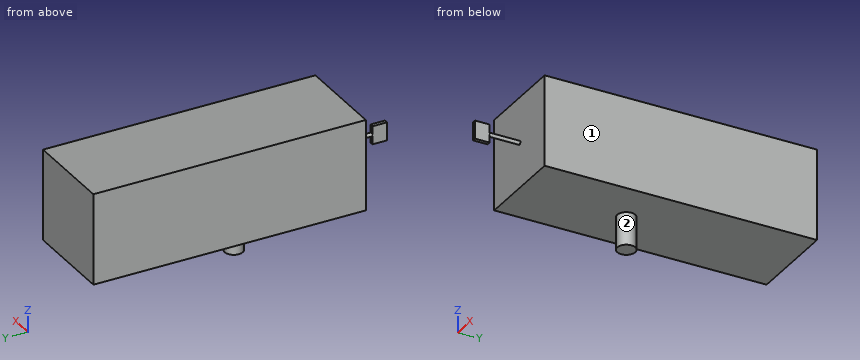
```python
from build123d import *

# Parameters (mm, degrees)
F0_W     = 50
F0_H     = 50
F1_DEPTH = 150
F2_R     = 1
F3_DEPTH = 25
F4_W     = 2
F4_H     = 10
F5_DEPTH = 8
F6_R     = 5
F7_DEPTH = 18


with BuildPart() as f1:
    # F0 (on Front) → F1 (new body)
    with BuildSketch(Plane.XZ):
        with Locations((0, 25)):
            Rectangle(F0_W, F0_H)
    extrude(amount=F1_DEPTH)

    # F2 (on face) → F3 (join)
    with BuildSketch(Plane.XZ.offset(150)):
        with Locations((0, 25)):
            Circle(F2_R)
    extrude(amount=F3_DEPTH)

    # F4 (on face) → F5 (join)
    with BuildSketch(Plane.XZ.offset(175)):
        with Locations((0, 25)):
            Rectangle(F4_W, F4_H)
    extrude(amount=-F5_DEPTH)

    # F6 (on face) → F7 (join)
    with BuildSketch(Plane(origin=(0, 0, 0), x_dir=(1, 0, 0), z_dir=(0, 0, -1))):
        with Locations((0, 91.149837)):
            Circle(F6_R)
    extrude(amount=F7_DEPTH)


solid = f1.part
```
Geometry check sheet. Reference: the model listing, model coordinates, mm. Face numbers are marked on the shaded views. A direction names the side the tool comes from. Coordinates: 2 decimals unless noted, no trailing zeros. Order: outer loops, then holes, each group sorted by start corner. A loop starts at its lowest first (then second) coordinate and runs counter-clockwise, first axis right, second up. Notation, with made-up numbers: (57.5, 64) - (108.5, 64) arc R20 ccw to (108.5, 84) - close; hole circle Ø4 at (47.25, 71.25). An arc over 180 degrees is marked (long way). Answer as a JSON object with one key per item and string values. Group by question number.
Item 1: Tool access check on the marked faces 1 and 2. Record the directions out of +Z, -Z, +X, -X, +Y, -Y that give a thin tool (end or side, any length) a straight path to the whole face; none if there is none.
Item 2: Sectioned sample at A-A, the plane x = -10. Record the cut outline in (y, z), and give its area (3 significant figures).
Item 3: Sectioned sample at B-B, the plane z = 38. Record the cut outline in (x, y).
Item 4: Scan lines: probe 1 along Y at (x, z) = (-12.5, 3); probe 2 along Z at (x, y) = (-4, -38); probe 3 along Y at (x, z) = (-2, -3). Record each from-to range of solid material in increasing order.
Item 5: Depth check by flat-ended pin: pin 1 Ø2.5 at (y, z) = (-172, 25) entering from -X; pin 2 Ø0.6 at (x, y) = (0, -171) entering from +Z; pin 3 Ø5 at (x, z) = (-6, 17) entering from -Y. Enter the tip coordinate at first touch or a pass-through.
Resolved:
{
 "1": {"face 1": "+Z, -Z, +X, +Y, -Y", "face 2": "-Z"},
 "2": {"outline": "(-150, 0) - (0, 0) - (0, 50) - (-150, 50) - close", "area": "7,500 mm^2"},
 "3": {"outline": "(-25, -150) - (25, -150) - (25, 0) - (-25, 0) - close"},
 "4": {"probe 1": "-150 to 0", "probe 2": "0 to 50", "probe 3": "-95.73 to -86.57"},
 "5": {"pin 1": "x = -1", "pin 2": "z = 30", "pin 3": "y = -150"}
}
